```python
from build123d import *

# Parameters (mm, degrees)
F1_DEPTH = 5.08


# Not quite as in the source:
# - a feature names something its author has since deleted; it is built from what else it names


with BuildPart() as f1:
    # F0 (on Front) → F1 (new body)
    with BuildSketch(Plane.XZ):
        Polygon((-25.4, 0), (0, 0), (25.4, 0), (25.4, -5.08), (63.5, -5.08), (63.5, 0), (88.9, 0), (88.9, 3.1722693238), (88.9, 6.3445386477), (88.9, 12.9838371649), (-88.9, 12.9838371649), (-88.9, 6.3445386477), (-88.9, 3.1722693238), (-88.9, 0), (-63.5, 0), (-63.5, -5.08), (-25.4, -5.08), align=None)
    extrude(amount=F1_DEPTH)


solid = f1.part
```
The listing builds one solid part. Answer for the finished solid, in the listing's coordinates (mm). A direction names the side the tool comes from. Round coordinates to 2 decimals unless told otherwise and drop trailing zeros. Loops run counter-clockwise (first coordinate to the right, second up) from the corner with the lowest first, then second, coordinate; pieces in that order, holes last. Notation, with made-up numbers: (33, 8) -> (61, 8) arc R20 cw to (61, 16) -> close; hole circle Ø9 at (2, 69.25). An arc over 180 degrees is marked (long way). Use one line per item in the form item = value.
1. Find the intervals of material crossed by probe 1 along X at (y, z) = (-4.5, -0.25); probe 2 along Z at (x, y) = (72.5, -4.2), in increasing order. Write a range as [from, to].
Answer key:
probe_1 = [-63.5, -25.4], [25.4, 63.5]
probe_2 = [0, 12.98]
2. A tool of negligible diameter and unlimited length cuts with its end or side. For faces 4 (the flat face through (76, -3, 0)), 5 (the flat face through (-45, -3, -5.08)), 6 (the flat face through (0, -3, 0)), 7 (the flat face through (-76, -3, 0)), 8 (the flat face through (1, -3, 12.984)), from which of +Z, -Z, +X, -X, +Y, -Y can it reach the whole face along a straight path? Write none if from no direction.
Answer key:
face_4 = -Z, +X, +Y, -Y
face_5 = -Z, +X, -X, +Y, -Y
face_6 = -Z, +Y, -Y
face_7 = -Z, -X, +Y, -Y
face_8 = +Z, +X, -X, +Y, -Y
3. Flat-ended cylindrical pins translate along their axes: pin 1 Ø1.5 at (x, y) = (76.5, -3) entering from -Z; pin 2 Ø1.5 at (y, z) = (-1.5, -3) entering from -X; pin 3 Ø1.5 at (y, z) = (-2.5, -1.5) entering from +X. Find the tip coordinate at first contact, or state that the pin passes through.
Answer key:
pin_1 = 0
pin_2 = -63.5
pin_3 = 63.5
4. The part is cut by section A-A on y = -3.1. Determine the outline of the cut face in (x, z).
Answer key:
outline = (-88.9, 0) -> (-63.5, 0) -> (-63.5, -5.08) -> (-25.4, -5.08) -> (-25.4, 0) -> (25.4, 0) -> (25.4, -5.08) -> (63.5, -5.08) -> (63.5, 0) -> (88.9, 0) -> (88.9, 12.98) -> (-88.9, 12.98) -> close
5. The part is cut by section B-B on x = 7. Determine the outline of the cut face in (y, z).
Answer key:
outline = (-5.08, 0) -> (0, 0) -> (0, 12.98) -> (-5.08, 12.98) -> close
6. For a pull along X with two mould halves and no side action, classify faces 1 (the flat face through (-1, -5.08, 4)), 2 (the flat face through (-25.4, -3, -3)), 3 (the flat face through (-63.5, -3, -3)) as released by +X, released by -X, zero draft, split by the parting line, or undercut.
Answer key:
face_1 = zero draft
face_2 = undercut
face_3 = released by -X
